```python
from build123d import *

# Parameters (mm, degrees)
SKETCH1_R           = 4
SKETCH1_R_2         = 2.5
BOSS_EXTRUDE1_DEPTH = 6
BOSS_EXTRUDE2_DEPTH = 2
CIRPATTERN1_COUNT   = 5


with BuildPart() as part:
    # Sketch1 → Boss-Extrude1 (new body)
    with BuildSketch(Plane(origin=(0, 0, 0), x_dir=(1, 0, 0), z_dir=(0, 1, 0))):
        Circle(SKETCH1_R)
        Circle(SKETCH1_R_2, mode=Mode.SUBTRACT)
    extrude(amount=BOSS_EXTRUDE1_DEPTH)

    # Sketch2 → Boss-Extrude2 (add)
    with BuildSketch(Plane(origin=(0, 6, 0), x_dir=(1, 0, 0), z_dir=(0, 1, 0))):
        with BuildLine():
            Line((-0.659397634, 3.945274992), (-0.659397634, 41.803919823))
            ThreePointArc((-0.659397634, 41.803919823), (4.137285492, 46.574729802), (8.882082768, 41.752313842))
            ThreePointArc((8.882082768, 41.752313842), (7.966424676, 27.945777977), (4.058060811, 14.672362658))
            ThreePointArc((4.058060811, 14.672362658), (2.118281369, 9.384999918), (0.659397634, 3.945274992))
            ThreePointArc((0.659397634, 3.945274992), (0, 4), (-0.659397634, 3.945274992))
        make_face()
    boss_extrude2 = extrude(amount=-BOSS_EXTRUDE2_DEPTH)

    # CirPattern1: Boss-Extrude2 ×5 about axis
    cirpattern1_axis = Axis((0, 0, 0), (0, 1, 0))
    for i in range(1, CIRPATTERN1_COUNT):
        add(boss_extrude2.rotate(cirpattern1_axis, i * 360 / CIRPATTERN1_COUNT))


solid = part.part
```
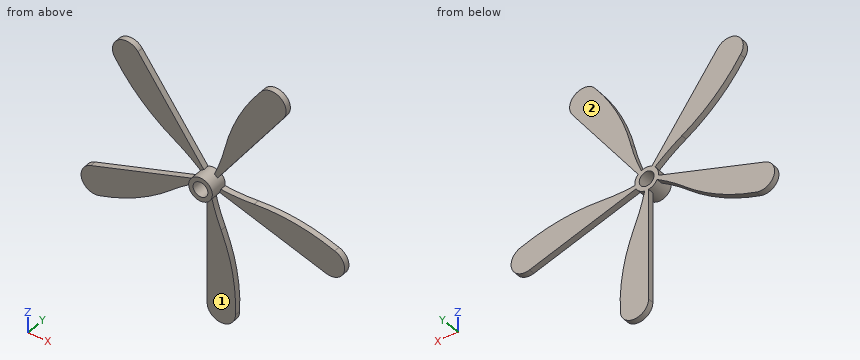
Design review of the part built by this model. Coordinates are the model's own, in mm. Face numbers are marked on the shaded views. A direction names the side the tool comes from. Coordinates: 2 decimals unless noted, no trailing zeros. Order: outer loops, then holes, each group sorted by start corner. A loop starts at its lowest first (then second) coordinate and runs counter-clockwise, first axis right, second up. Notation, with made-up numbers: (42, 74) -> (62, 74) arc R26 cw to (62, 95) -> close; hole circle Ø9 at (89, 50.5). An arc over 180 degrees is marked (long way). One line per item, written item: value. Start each with the question number.
Q1. Insertion check: pin 1 Ø3 at (x, z) = (3.5, -33) entering from -Y; pin 2 Ø1.6 at (y, z) = (5.5, -18.5) entering from -X; pin 3 Ø1.5 at (y, z) = (4.5, 10.5) entering from -X; pin 4 Ø6 at (x, z) = (-33.5, 23.5) entering from +Y. Each pin has a flat end and moves straight along its axis. Give the tip position at first contact, or say it passes through.
Q2. Take a section at C-C, the plane y = 2.2. State the section outline as (x, z) points, then the cut area to 3 significant figures.
Q3. Tool access review of the marked faces 1 and 2: name each direction out of +Z, -Z, +X, -X, +Y, -Y from which nothing blocks a thin tool from reaching the whole face with its end or side.
Q4. For probe 1 along X at (y, z) = (2, 0); probe 2 along Y at (x, z) = (-21.5, 19), list the stretches that pass through material, from the lowest coordinate up.
Q5. Take a section at B-B, the plane z = 11.5. State the section outline as (x, y) points.
Q6. Take a section at D-D, the plane x = 32.5. State the section outline as (y, z) points.
Q7. Take a section at A-A, the plane x = -19. State the section outline as (y, z) points.
Values follow:
1. pin 1: stops at y = 4
1. pin 2: stops at x = -43.18
1. pin 3: stops at x = -14.65
1. pin 4: passes through
2. outline: circle Ø8 at (0, 0); hole circle Ø5 at (0, 0)
2. area: 30.6 mm2
3. face 1: -Z, +X, -X, -Y
3. face 2: +Z, -Z, +X, -X, +Y
4. probe 1: x = -4 to -2.5, 2.5 to 4
4. probe 2: y = 4 to 6
5. outline: (-15.01, 4) -> (-7.54, 4) -> (-7.54, 6) -> (-15.01, 6) -> close; (4.62, 4) -> (9.17, 4) -> (9.17, 6) -> (4.62, 6) -> close
6. outline: (4, -11.25) -> (6, -11.25) -> (6, -1.64) -> (4, -1.64) -> close
7. outline: (4, -13.16) -> (6, -13.16) -> (6, -5.48) -> (4, -5.48) -> close; (4, 14.5) -> (6, 14.5) -> (6, 27.27) -> (4, 27.27) -> close
